Geometry check sheet. Reference: drawing and pictorial views, mm from the part's lowest x, y, z. A direction names the side the tool comes from. Give positions to 0.01 mm unless a question says otherwise; leave off trailing zeros. Order: outer loops, then holes, each group sorted by start corner. A loop starts at its lowest first (then second) coordinate and runs counter-clockwise, first axis right, second up. Notation, with made-up numbers: (-8.5, 83) -> (34.5, 83) arc R27 ccw to (34.5, 105) -> close; hole circle Ø2 at (44.25, -3). An arc over 180 degrees is marked (long way). Write each question's results on one line, items separated by ' | '. Start each with the question number.
1. Cross-section at D-D, the plane z = 1.5. Enter the section's corners in (x, y).
2. Mould release check, pull along X, two halves, no side actions. Record for the marked faces 1, 2 and 3: +X half, -X half, draft (parallel to the pull), parting line (faces both ways), or undercut.
3. Cross-section at C-C, the plane x = 52. Enter the section's corners in (y, z), then the cut area to 3 significant figures.
4. Depth check by flat-ended pin: pin 1 Ø2 at (y, z) = (33, 11.5) entering from +X; pin 2 Ø0.7 at (y, z) = (1.5, 6.5) entering from -X; pin 3 Ø4 at (x, y) = (30, 38.5) entering from -Z; pin 4 Ø5.5 at (y, z) = (53.5, 8.5) entering from -X. Enter the tip coordinate at first touch or a pass-through.
5. Material ranges on L1, parallel to X at y = 5, z = 9.5; L2, parallel to Y at x = 52, z = 17.6; L3, parallel to X at y = 13.5, z = 9.5 (1 decimal), recorded low to high. Write a range as from..to.
6. Set-up check for the marked faces 4, 5 and 6: record each of +Z, -Z, +X, -X, +Y, -Y from which the full face is reachable in a straight line by a thin tool's end or side.
7. Cross-section at A-A, the plane z = 9.5. Enter the section's corners in (x, y).
8. Cross-section at B-B, the plane y = 35. Enter the section's corners in (x, z), then the cut area to 3 significant figures.
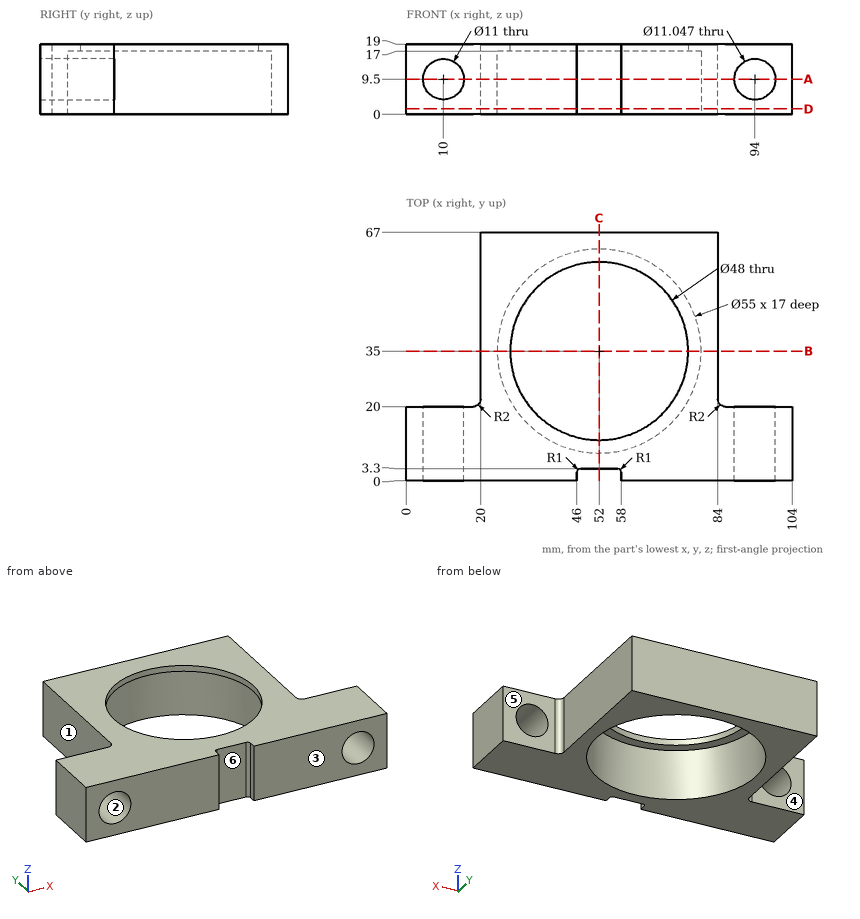
Results below:
1) outline: (0, 0) -> (46, 0) -> (46, 2.3) arc R1 cw to (47, 3.3) -> (57, 3.3) arc R1 cw to (58, 2.3) -> (58, 0) -> (104, 0) -> (104, 20) -> (86, 20) arc R2 cw to (84, 22) -> (84, 67) -> (20, 67) -> (20, 22) arc R2 cw to (18, 20) -> (0, 20) -> close; hole circle Ø55 at (52, 35)
2) face 1: -X half | face 2: undercut | face 3: draft
3) outline: (3.3, 0) -> (7.5, 0) -> (7.5, 17) -> (11, 17) -> (11, 19) -> (3.3, 19) -> close; (59, 17) -> (62.5, 17) -> (62.5, 0) -> (67, 0) -> (67, 19) -> (59, 19) -> close | area: 179 mm²
4) pin 1: stops at x = 84 | pin 2: stops at x = 0 | pin 3: stops at z = 17 | pin 4: stops at x = 20
5) L1: x = 0..4.5, 15.5..88.48, 99.52..104 | L2: y = 3.3..11, 59..67 | L3: x = 0..4.5, 15.5..34.9, 69.1..88.5, 99.5..104
6) face 4: +Z, -Z, -X, +Y | face 5: +Z, -Z, +X, +Y | face 6: +Z, -Z, -Y
7) outline: (0, 0) -> (4.5, 0) -> (4.5, 20) -> (0, 20) -> close; (15.5, 0) -> (46, 0) -> (46, 2.3) arc R1 cw to (47, 3.3) -> (57, 3.3) arc R1 cw to (58, 2.3) -> (58, 0) -> (88.48, 0) -> (88.48, 20) -> (86, 20) arc R2 cw to (84, 22) -> (84, 67) -> (20, 67) -> (20, 22) arc R2 cw to (18, 20) -> (15.5, 20) -> close; (99.52, 0) -> (104, 0) -> (104, 20) -> (99.52, 20) -> close; hole circle Ø55 at (52, 35)
8) outline: (20, 0) -> (24.5, 0) -> (24.5, 17) -> (28, 17) -> (28, 19) -> (20, 19) -> close; (76, 17) -> (79.5, 17) -> (79.5, 0) -> (84, 0) -> (84, 19) -> (76, 19) -> close | area: 185 mm²
